from build123d import *

# Parameters (mm, degrees)
HEXDRIVE_DEPTH = 3


with BuildPart() as part:
    # BodySketch → Base-Revolve (revolve)
    with BuildSketch(Plane(origin=(0, 0, 0), x_dir=(1, 0, 0), z_dir=(0, 1, 0)), mode=Mode.PRIVATE) as base_revolve_sk:
        Polygon((-6, 0), (-6, 5), (0, 5), (0, 3), (19.4455, 3), (20, 2.4455), (20, 0), align=None)
    revolve(base_revolve_sk.sketch.rotate(Axis((-6, 0, 0), (1, 0, 0)), 180), axis=Axis((-6, 0, 0), (1, 0, 0)))

    # DriveSketch → HexDrive (cut)
    with BuildSketch(Plane.ZY.offset(6)):
        Polygon((2.898298351, 0), (1.449149176, 2.51), (-1.449149176, 2.51), (-2.898298351, 0), (-1.449149176, -2.51), (1.449149176, -2.51), align=None)
    extrude(amount=-HEXDRIVE_DEPTH, mode=Mode.SUBTRACT)


solid = part.part
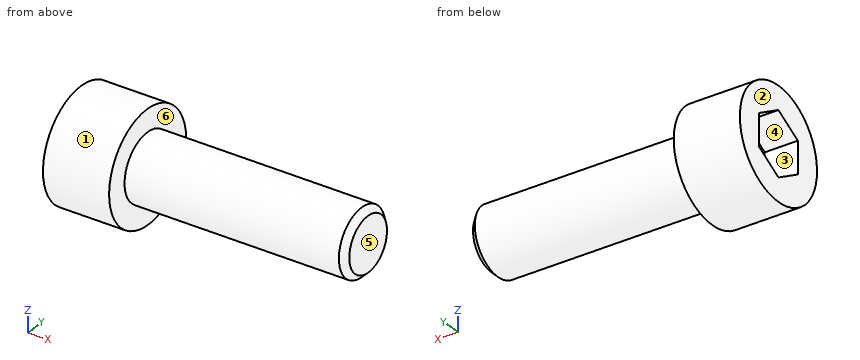
Here's how the part is built. I have some questions about the finished solid (model axes, mm). Face numbers are marked on the shaded views. A direction names the side the tool comes from. Round coordinates to 2 decimals unless told otherwise and drop trailing zeros. Order: outer loops, then holes, each group sorted by start corner. A loop starts at its lowest first (then second) coordinate and runs counter-clockwise, first axis right, second up. Notation, with made-up numbers: (53, 63) -> (103, 63) arc R36 cw to (103, 102) -> close; hole circle Ø4 at (-18, -14). An arc over 180 degrees is marked (long way). Use CSV: the item, a comma, the result in double quotes.
1. Thinking about a two-plate mould opening in Z: for the marked faces 1, 2 and 3, which applies, pulls with the +Z half, pulls with the -Z half, needs draft (parallel to the pull), parting line crosses it, or undercut?
Recorded:
face 1,"parting line crosses it"
face 2,"needs draft"
face 3,"undercut"
2. I'm going to push flat-ended pins straight in: P1, Ø3, axis at x = 1, z = -2.5, coming from the +Y side; P2, Ø4, axis at y = 1, z = -0.5, coming from the -X side; P3, Ø4, axis at x = 1, y = -3, coming from the +Z side; P4, Ø1, axis at x = -2, y = -1, coming from the -Z side. Where does each tip first touch, or does it pass through?
Recorded:
P1,"stops at y = 4.81"
P2,"stops at x = -6"
P3,"stops at z = 4.84"
P4,"stops at z = -4.97"
3. I want a section at C-C on y = 3.25. List the corners of the cut face in (x, z) for me, and give its area (3 significant figures).
Recorded:
outline,"(-6, -3.8) -> (0, -3.8) -> (0, 3.8) -> (-6, 3.8) -> close"
area,"45.6 mm2"
4. I need wall thicknesses on line 1 along X through (y, z) = (-1.5, -0.5); line 2 along X through (y, z) = (4, 0.5); line 3 along Y through (x, z) = (10, 1.25). Which ranges of each line are inside material? Lowest first, please.
Recorded:
line 1,"x = -3 to 20"
line 2,"x = -6 to 0"
line 3,"y = -2.73 to 2.73"
5. Which directions (+Z, -Z, +X, -X, +Y, -Y) give clear straight access to the entire face, cutting with the end or side of a thin tool? Please do the marked faces 4, 5 and 6.
Recorded:
face 4,"-X"
face 5,"+Z, -Z, +X, +Y, -Y"
face 6,"+X"
6. I want a section at B-B on x = 15.5. List the corners of the cut face in (y, z) for me.
Recorded:
outline,"circle Ø6 at (0, 0)"
7. I want a section at A-A on z = 0. List the corners of the cut face in (x, y) for me.
Recorded:
outline,"(-6, -5) -> (0, -5) -> (0, -3) -> (19.45, -3) -> (20, -2.45) -> (20, 2.45) -> (19.45, 3) -> (0, 3) -> (0, 5) -> (-6, 5) -> (-6, 2.51) -> (-3, 2.51) -> (-3, -2.51) -> (-6, -2.51) -> close"
